Autodesk Inventor part; units mm, degrees
ref_plane "Work Plane1" through (30, 0, 0) normal (0, -0.5, 0.866) x (1, 0, 0)
ref_plane "YZ Plane" through (0, 0, 0) normal (1, 0, 0) x (0, 1, 0)
ref_plane "XZ Plane" through (0, 0, 0) normal (0, 1, 0) x (-1, 0, 0)
sketch "Sketch1" plane through (0, 0, 0) normal (0, 0, 1) x (1, 0, 0)
  line L0 (0.1133, 0) -> (16, 0)
  line L1 (16, 0) -> (16, 3)
  line L2 (16, 3) -> (2, 3)
  line L3 (2, 3) -> (1.3865, 3)
  line L4 (1.3865, 3) -> (0, 3)
  line L5 (0, 3) -> (0, 5.25)
  line L6 (0, 5.25) -> (-3.3, 5.25)
  line L7 (-3.3, 5.25) -> (-3.3, 2.3094)
  line L8 (-3.3, 2.3094) -> (-1.22, 2.3094)
  line L9 (-1.22, 2.3094) -> (0.1133, 0)
  line L10 (-7.16, 0) -> (19.86, 0)
  line L11 (0, -1.05) -> (0, 6.3)
  line L12 (2, 3) -> (0, 3) construction
  dimension "d0" = 14
  dimension "d1" = 0.6135
  dimension "d2" = 3.3
  dimension "d3" = 2.08
  dimension "d4" = 60
  dimension "d5" = 6
  dimension "d6" = 6
  dimension "d7" = 4.6188
  dimension "d8" = 10.5
  dimension "d19" = 16
revolve "Body" add sketch "Sketch1" angle 360 about axis through (0.1133, 0, 0) along (1, 0, 0) contours L9 L11 L4 L3 L2 L1 L0 | L9 L8 L7 L6 L5 L11
sketch "Sketch2" plane through (-3.3, 0, 0) normal (-1, 0, 0) x (0, 0, 1)
  circle A0 centre (0, 0) radius 2.3094
  line L0 (0, -7.35) -> (0, 7.35)
  line L1 (-7.35, 0) -> (7.35, 0)
  line L2 (2.3094, 0) -> (1.1547, -2)
  line L3 (1.1547, -2) -> (-1.1547, -2)
  line L4 (-1.1547, -2) -> (-2.3094, 0)
  line L5 (-2.3094, 0) -> (-1.1547, 2)
  line L6 (-1.1547, 2) -> (1.1547, 2)
  line L7 (1.1547, 2) -> (2.3094, 0)
extrude "Slot" add sketch "Sketch2" against normal up to next contours L7 A0 | A0 L2 | L6 L0 A0 | A0 L0 L3 | L0 L6 A0 | A0 L3 L0 | L4 A0 | A0 L5
fillet "Fillet1" radius 2.625 1 edges at (-3.3, -5.25, 0)
thread "Thread"
chamfer "Chamfer1" distance 0.6135 distance2 0.6135 1 edges at (16, -3, 0) measured on face at (16, -1.1424, 0.935)
fillet "Fillet2" radius 0.25 1 edges at (0, -3, 0)
ref_plane "Work Plane1" through (30, 0, 0) normal (0, -0.5, 0.866) x (1, 0, 0)
equation "\"d0\" = GEL"
equation "\"d1\" = GAL"
equation "\"d2\" = KOH"
equation "\"d3\" = INTI"
equation "\"d5\" = GD"
equation "\"d6\" = BDM"
equation "\"d7\" = 1.1547 * SW"
equation "\"d8\" = KOD"
equation "\"d19\" = NLG"
equation "\"d16\" = RR"
equation "\"d12\" = GEL"
equation "\"d14\" = -0.5 * SPD + 0.5 * GD"
equation "\"d15\" = GUL"
equation "\"d29\" = R"
equation "\"GD\" = NND"
equation "\"NLG\" = 16"
equation "\"GEL\" = 14"
equation "\"KOD\" = 10.5"
equation "\"KOH\" = 3.3"
equation "\"INTI\" = 2.08"
equation "\"GAL\" = 0.61345 * PTC"
equation "\"GUL\" = 0.61345 * PTC"
equation "\"BDM\" = NND"
equation "\"SW\" = 4"
equation "\"RR\" = 2.625"
equation "\"SPD\" = 4.7731"
equation "\"d28\" = R"
equation "\"R\" = 0.25"
equation "\"TOA\" = 30deg"
equation "\"THREADDIA\" = 6"
equation "\"KOD1\" = KOD - 2 * RR"
equation "\"PTC\" = 1"
equation "\"NND\" = 6"
equation "\"E0\" = 1.155 * SW"
equation "\"GD1\" = THREADDIA - 1.2269 * PTC"
properties part number "PWTR-0105" material "Steel, Mild"
Input: part model. Units: mm. Frame: model coordinates. A direction names the side the tool comes from. Give positions to 0.01 mm unless a question says otherwise; leave off trailing zeros. Loops run counter-clockwise (first coordinate to the right, second up) from the corner with the lowest first, then second, coordinate; pieces in that order, holes last. Notation, with made-up numbers: (43, 77) -> (83, 77) arc R27 ccw to (83, 113) -> close; hole circle Ø3 at (21.5, -36). An arc over 180 degrees is marked (long way). Answer as a JSON object with one key per item and string values. Group by question number.
Item 1: Pin query (flat end, axial travel): P1, Ø0.7, axis at x = -2, z = 0.5, coming from the -Y side; P2, Ø3, axis at y = -2.5, z = -1.5, coming from the +X side; P3, Ø3, axis at x = 8.5, z = 3, coming from the +Y side; P4, Ø3, axis at x = 3.5, y = -2.5, coming from the -Z side. Return the tip coordinate at first contact, or that it passes through.
Item 2: Reachability of faces 5 (the flat face through (16, 0, 0)), 6 (the flat face through (0, -0.1, -3.4)), 7 (the flat face through (-2.19, 0.99, -1.74)) from +Z, -Z, +X, -X, +Y, -Y: full face, straight path, thin tool, end or side. Return the list, or none.
Item 3: Cut plane A-A, the plane x = 3. Return the cut outline in (y, z), and give its area (3 significant figures).
Item 4: Line query: probe 1 along Y at (x, z) = (-2.25, 0.5); probe 2 along Y at (x, z) = (10.75, -1); probe 3 along Y at (x, z) = (12, -2.25). Output: solid intervals per line, ascending.
Item 5: Pull-direction query (Y, two-part tool) for faces 1 (the cylindrical face through (-0.3, 5, -1.6)), 2 (the flat face through (-2.19, -0.99, 1.74)), 3 (the flat face through (-2.186, -1.014, -1.724)), 4 (the flat face through (-3.3, -1, -2)); classes: released by +Y, released by -Y, zero draft, split by the parting line, or undercut.
Checks:
{
 "1": {"P1": "stops at y = -5.04", "P2": "stops at x = 16", "P3": "stops at y = 2.6", "P4": "stops at z = -2.83"},
 "2": {"face 5": "+Z, -Z, +X, +Y, -Y", "face 6": "+X", "face 7": "-X"},
 "3": {"outline": "circle Ø6 at (0, 0)", "area": "28.3 mm²"},
 "4": {"probe 1": "y = -4.7 to -2, 2 to 4.7", "probe 2": "y = -2.83 to 2.83", "probe 3": "y = -1.98 to 1.98"},
 "5": {"face 1": "split by the parting line", "face 2": "undercut", "face 3": "undercut", "face 4": "zero draft"}
}
